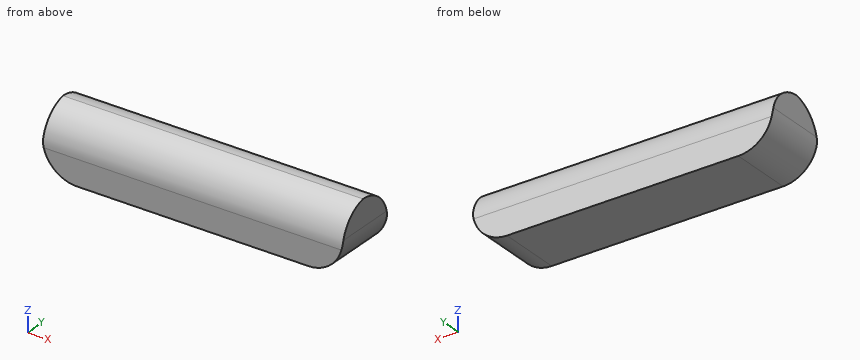
from build123d import *

# Parameters (mm, degrees)
F0_W        = 49.567822367
F0_H        = 20.8045206964
F1_DEPTH    = 20
F2_R        = 11.3468037432
F3_T1_DEPTH = 107.5148856448
F4_R        = 11.3468037432


# Not quite as in the source:
# - a fillet or chamfer that OpenCascade refuses, or shapes differently, is made with other operations: its cross-section is extruded or revolved along the edge and cut away or added


with BuildPart() as f1:
    # F0 (on Top) → F1 (new body)
    with BuildSketch(Plane.XY):
        with Locations((-24.7839111835, -10.4022603482)):
            Rectangle(F0_W, F0_H)
    extrude(amount=F1_DEPTH)

    # F2
    f2_edges = [f1.edges().sort_by_distance(p)[0] for p in [
        (-24.783911, 0, 20),
    ]]
    fillet(f2_edges, radius=F2_R)

    # F3: fillet of radius 11.8296464556 on 1 edges, made by hand

    # F3_s2 → F3_t1 (cut)
    with BuildSketch(Plane.YZ.offset(-78.5413540059)):
        with BuildLine():
            ThreePointArc((-11.3468037432, 20), (-18.1400153389, 15.8899405195), (-20.8045206964, 8.4105873444))
            Line((-20.8045206964, 8.4105873444), (-20.8045206964, 20))
            Line((-20.8045206964, 20), (-11.3468037432, 20))
        make_face()
    extrude(amount=F3_T1_DEPTH, mode=Mode.SUBTRACT)

    # F4
    f4_edges = [f1.edges().sort_by_distance(p)[0] for p in [
        (-49.567822, -10.40226, 0),
    ]]
    fillet(f4_edges, radius=F4_R)

    # F5: F1 across face


with BuildPart() as f1_1:
    add(f1.part)
    add(f1.part.mirror(Plane(origin=(0, -10.3947828822, 8.8652235267), x_dir=(0, 1, 0), z_dir=(1, 0, 0))))


solid = f1_1.part
Geometry check sheet. Reference: the model listing, model coordinates, mm. Coordinates: 2 decimals unless noted, no trailing zeros. Write each loop counter-clockwise with the first axis right and the second up, starting at its lowest first coordinate (ties: lowest second). Pieces come first, ordered by that corner, then holes. Notation, with made-up numbers: (36.5, 38) -> (43.5, 38) arc R19 cw to (43.5, 61) -> close; hole circle Ø2 at (70.25, -38). An arc over 180 degrees is marked (long way). One line per question, with ' | ' between items.
1. Thickness scan on probe 1 along X at (y, z) = (-10, 10.75); probe 2 along Y at (x, z) = (3, 16.5); probe 3 along X at (y, z) = (-9.75, 1). Record the ranges inside material, lowest first. Write a range as from..to.
Answers:
probe 1: x = -49.55..49.55 | probe 2: y = -17.61..-3.15 | probe 3: x = -42.88..42.88
2. Cross-section at C-C on z = 5.75. Record the cut outline in (x, y).
Answers:
outline: (-48.09, -20.8) -> (48.09, -20.8) -> (48.09, 0) -> (-48.09, 0) -> close
3. Cross-section at B-B on y = -8.5. Record the cut outline in (x, z).
Answers:
outline: (-49.57, 11.35) arc R11.35 ccw to (-38.22, 0) -> (38.22, 0) arc R11.35 ccw to (49.57, 11.35) -> (49.57, 19.64) -> (-49.57, 19.64) -> close
4. Cross-section at A-A on x = 12. Record the cut outline in (y, z), and give its area (3 significant figures).
Answers:
outline: (-20.8, 0) -> (0, 0) -> (0, 8.65) arc R11.35 ccw to (-11.35, 20) arc R11.83 ccw to (-20.8, 8.41) -> close | area: 361 mm²
5. Depth check by flat-ended pin: pin 1 Ø8 at (x, z) = (-1.5, 13.5) entering from -Y; pin 2 Ø10 at (y, z) = (-9, 2.5) entering from +X; pin 3 Ø1.5 at (x, z) = (25, 13.5) entering from +Y. Enter the tip coordinate at first touch or a pass-through.
Answers:
pin 1: stops at y = -20.75 | pin 2: stops at x = 48.9 | pin 3: stops at y = -0.77
6. Cross-section at D-D on y = -2. Record the cut outline in (x, z), and give its area (3 significant figures).
Answers:
outline: (-49.57, 11.35) arc R11.35 ccw to (-38.22, 0) -> (38.22, 0) arc R11.35 ccw to (49.57, 11.35) -> (49.57, 15.09) -> (-49.57, 15.09) -> close | area: 1,440 mm²
